```python
from build123d import *

# Parameters (mm, degrees)
SKETCH1_R           = 4.75
BOSS_EXTRUDE1_DEPTH = 87
SKETCH2_R           = 17.25
BOSS_EXTRUDE2_DEPTH = 4
SKETCH3_R           = 5
CUT_EXTRUDE1_DEPTH  = 4
BOSS_EXTRUDE3_START = 6.5
SKETCH4_W           = 3.5
SKETCH4_H           = 6.777720856
BOSS_EXTRUDE3_DEPTH = 9
BOSS_EXTRUDE4_START = 41.5
SKETCH5_W           = 3.5
SKETCH5_H           = 6.777720856
BOSS_EXTRUDE4_DEPTH = 5


with BuildPart() as part:
    # Sketch1 → Boss-Extrude1 (new body)
    with BuildSketch(Plane(origin=(0, 0, 0), x_dir=(1, 0, 0), z_dir=(0, 1, 0))):
        with Locations(Location((0, 0, 0), (0, 0, 270))):
            Circle(SKETCH1_R)
    extrude(amount=BOSS_EXTRUDE1_DEPTH)

    # Sketch2 → Boss-Extrude2 (add)
    with BuildSketch(Plane(origin=(0, 0, 0), x_dir=(-1, 0, 0), z_dir=(0, -1, 0))):
        with Locations(Location((0, 0, 0), (0, 0, 90))):
            Circle(SKETCH2_R)
    extrude(amount=BOSS_EXTRUDE2_DEPTH)

    # Sketch3 → Cut-Extrude1 (cut)
    with BuildSketch(Plane.XZ.offset(4)):
        with Locations(Location((0, 10, 0), (0, 0, 270))):
            Circle(SKETCH3_R)
    extrude(amount=-CUT_EXTRUDE1_DEPTH, mode=Mode.SUBTRACT)

    # Sketch4 → Boss-Extrude3 (add)
    with BuildSketch(Plane(origin=(0, 0, 0), x_dir=(1, 0, 0), z_dir=(0, 1, 0)).offset(BOSS_EXTRUDE3_START)):
        with Locations((0, 3.388860428)):
            Rectangle(SKETCH4_W, SKETCH4_H)
    extrude(amount=BOSS_EXTRUDE3_DEPTH)

    # Sketch5 → Boss-Extrude4 (add)
    with BuildSketch(Plane(origin=(0, 0, 0), x_dir=(1, 0, 0), z_dir=(0, 1, 0)).offset(BOSS_EXTRUDE4_START)):
        with Locations((0, 3.388860428)):
            Rectangle(SKETCH5_W, SKETCH5_H)
    extrude(amount=BOSS_EXTRUDE4_DEPTH)


solid = part.part
```
Work out the finished part from the listing and answer in its coordinate system (mm). A direction names the side the tool comes from. Give positions to 0.01 mm unless a question says otherwise; leave off trailing zeros. Order: outer loops, then holes, each group sorted by start corner. A loop starts at its lowest first (then second) coordinate and runs counter-clockwise, first axis right, second up. Notation, with made-up numbers: (46.5, 41.5) - (97.5, 41.5) arc R29 ccw to (97.5, 75.5) - close; hole circle Ø7 at (66.5, 39.5). An arc over 180 degrees is marked (long way). One line per item, written item: value. Start each with the question number.
1. Section A-A, the plane x = 0 is taken. Write down the section's boundary in (y, z), then the cut area to 3 significant figures.
2. For a pull along X with two mould halves and no side action, classify faces 1 (the face through (1.5, -2.03, 5.23)), 2 (the face through (0, 11, -6.778)), 3 (the face through (-1.75, 11, -6)) as released by +X, released by -X, zero draft, split by the parting line, or undercut.
3. Section C-C, the plane z = 10 is taken. Write down the section's boundary in (x, y).
4. Consider line 1 (Y direction, x = -2.5, z = -14); line 2 (X direction, y = -1, z = 10); line 3 (X direction, y = 75.5, z = -3). Determine where each line is inside the solid, lowest interval first.
5. Each of these flat-tipped pins is pushed along its axis until it touches: pin 1 Ø0.7 at (x, z) = (1, -5.5) entering from +Y; pin 2 Ø2.5 at (y, z) = (11, -6) entering from -X; pin 3 Ø8 at (x, y) = (1, 25) entering from -Z. Where does it stop, or does it pass through?
6. Section D-D, the plane y = 18 is taken. Write down the section's boundary in (x, z), then the cut area to 3 significant figures.
7. Section B-B, the plane z = 0 is taken. Write down the section's boundary in (x, y).
8. Which of the six approach directions +Z, -Z, +X, -X, +Y, -Y give full straight-line access (tool end or side, diameter ignored) to faces 4 (the face through (-1.75, 44, -6)), 5 (the face through (1.75, 11, -6)), 6 (the face through (0, 44, -6.778))?
Filled sheet:
1. outline: (-4, -17.25) - (0, -17.25) - (0, -4.75) - (6.5, -4.75) - (6.5, -6.78) - (15.5, -6.78) - (15.5, -4.75) - (41.5, -4.75) - (41.5, -6.78) - (46.5, -6.78) - (46.5, -4.75) - (87, -4.75) - (87, 4.75) - (0, 4.75) - (0, 5) - (-4, 5) - close; (-4, 15) - (0, 15) - (0, 17.25) - (-4, 17.25) - close
1. area: 953 mm²
2. face 1: undercut
2. face 2: zero draft
2. face 3: released by -X
3. outline: (-14.06, -4) - (-5, -4) - (-5, 0) - (-14.06, 0) - close; (5, -4) - (14.06, -4) - (14.06, 0) - (5, 0) - close
4. line 1: -4 to 0
4. line 2: -14.06 to -5, 5 to 14.06
4. line 3: -3.68 to 3.68
5. pin 1: y = 46.5
5. pin 2: x = -1.75
5. pin 3: z = -4.75
6. outline: circle Ø9.5 at (0, 0)
6. area: 70.9 mm²
7. outline: (-17.25, -4) - (17.25, -4) - (17.25, 0) - (4.75, 0) - (4.75, 87) - (-4.75, 87) - (-4.75, 0) - (-17.25, 0) - close
8. face 4: -Z, -X, +Y
8. face 5: -Z, +X, +Y
8. face 6: -Z, +X, -X, +Y
